from build123d import *

# Parameters (mm, degrees)
F1_DEPTH = 10


with BuildPart() as f1:
    # F0 (on Front) → F1 (new body)
    with BuildSketch(Plane.XZ):
        with BuildLine():
            Line((-10, 0), (-25, 0))
            ThreePointArc((-25, 0), (-23.096988, -9.567086), (-17.67767, -17.67767))
            Line((-17.67767, -17.67767), (-7.071068, -7.071068))
            ThreePointArc((-7.071068, -7.071068), (-3.826834, -9.238795), (0, -10))
            Line((0, -10), (0, -25))
            ThreePointArc((0, -25), (9.567086, -23.096988), (17.67767, -17.67767))
            Line((17.67767, -17.67767), (7.071068, -7.071068))
            ThreePointArc((7.071068, -7.071068), (9.238795, -3.826834), (10, 0))
            Line((10, 0), (25, 0))
            ThreePointArc((25, 0), (23.096988, 9.567086), (17.67767, 17.67767))
            Line((17.67767, 17.67767), (7.071068, 7.071068))
            ThreePointArc((7.071068, 7.071068), (3.826834, 9.238795), (0, 10))
            Line((0, 10), (0, 25))
            ThreePointArc((0, 25), (-9.567086, 23.096988), (-17.67767, 17.67767))
            Line((-17.67767, 17.67767), (-7.071068, 7.071068))
            ThreePointArc((-7.071068, 7.071068), (-9.238795, 3.826834), (-10, 0))
        make_face()
    extrude(amount=F1_DEPTH)


solid = f1.part
Design review of the part built by this model. Coordinates are the model's own, in mm. A direction names the side the tool comes from. Coordinates: 2 decimals unless noted, no trailing zeros. Order: outer loops, then holes, each group sorted by start corner. A loop starts at its lowest first (then second) coordinate and runs counter-clockwise, first axis right, second up.
Item 1: The part is to be moulded in two halves that separate along Z. For faces 5 (the cylindrical face through (-23.15, -4.93, -9.44)), 6 (the flat face through (-17, -5, 0)), 7 (the flat face through (12, -5, 12)), say which applies: pulls with the +Z half, pulls with the -Z half, needs draft (parallel to the pull), parting line crosses it, or undercut.
Item 2: For faces 1 (the cylindrical face through (-9.218, -4.93, 3.878)), 2 (the flat face through (17, -5, 0)), 3 (the flat face through (0, -5, 17)), 4 (the flat face through (0, -5, -17)), list the 3-axis set-ups (+Z, -Z, +X, -X, +Y, -Y) from which the entire face can be reached by the end or side of a thin tool; tool diameter is ignored.
Item 3: Take a section at C-C, the plane z = 11. Write out the cut boundary in (x, y).
Item 4: For line 1 (Z direction, x = 12, y = -2.5); line 2 (X direction, y = -2.25, z = 15); line 3 (Z direction, x = 8.5, y = -8.5), list the stretches that pass through material, from the lowest coordinate up.
Item 5: Take a section at B-B, the plane y = -4.5. Write out the cut boundary in (x, z), then the cut area to 3 significant figures.
Item 6: For pin 1 Ø3 at (y, z) = (-4, 5) entering from +X; pin 2 Ø1.5 at (x, y) = (10, -8) entering from +Z; pin 3 Ø1 at (y, z) = (-2, 6.5) entering from -X, all flat-tipped, find the tip position at first contact; note any pin that passes through.
Item 7: Take a section at A-A, the plane x = 15. Write out the cut boundary in (y, z).
Item 8: Take a section at D-D, the plane z = 20. Write out the cut boundary in (x, y).
The answers:
1. face 5: pulls with the -Z half
1. face 6: undercut
1. face 7: pulls with the +Z half
2. face 1: -X, +Y, -Y
2. face 2: +X, +Y, -Y
2. face 3: +Z, +Y, -Y
2. face 4: -Z, +Y, -Y
3. outline: (-11, -10) - (0, -10) - (0, 0) - (-11, 0) - close; (11, -10) - (22.45, -10) - (22.45, 0) - (11, 0) - close
4. line 1: z = -21.93 to -12, 0 to 12
4. line 2: x = -15 to 0, 15 to 20
4. line 3: z = -23.51 to -8.5, -5.27 to 8.5
5. outline: (-25, 0) arc R25 ccw to (-17.68, -17.68) - (-7.07, -7.07) arc R10 ccw to (0, -10) - (0, -25) arc R25 ccw to (17.68, -17.68) - (7.07, -7.07) arc R10 ccw to (10, 0) - (25, 0) arc R25 ccw to (17.68, 17.68) - (7.07, 7.07) arc R10 ccw to (0, 10) - (0, 25) arc R25 ccw to (-17.68, 17.68) - (-7.07, 7.07) arc R10 ccw to (-10, 0) - close
5. area: 1,140 mm2
6. pin 1: stops at x = 24.75
6. pin 2: stops at z = 10.75
6. pin 3: stops at x = -8
7. outline: (-10, -20) - (0, -20) - (0, -15) - (-10, -15) - close; (-10, 0) - (0, 0) - (0, 15) - (-10, 15) - close
8. outline: (-15, -10) - (0, -10) - (0, 0) - (-15, 0) - close
